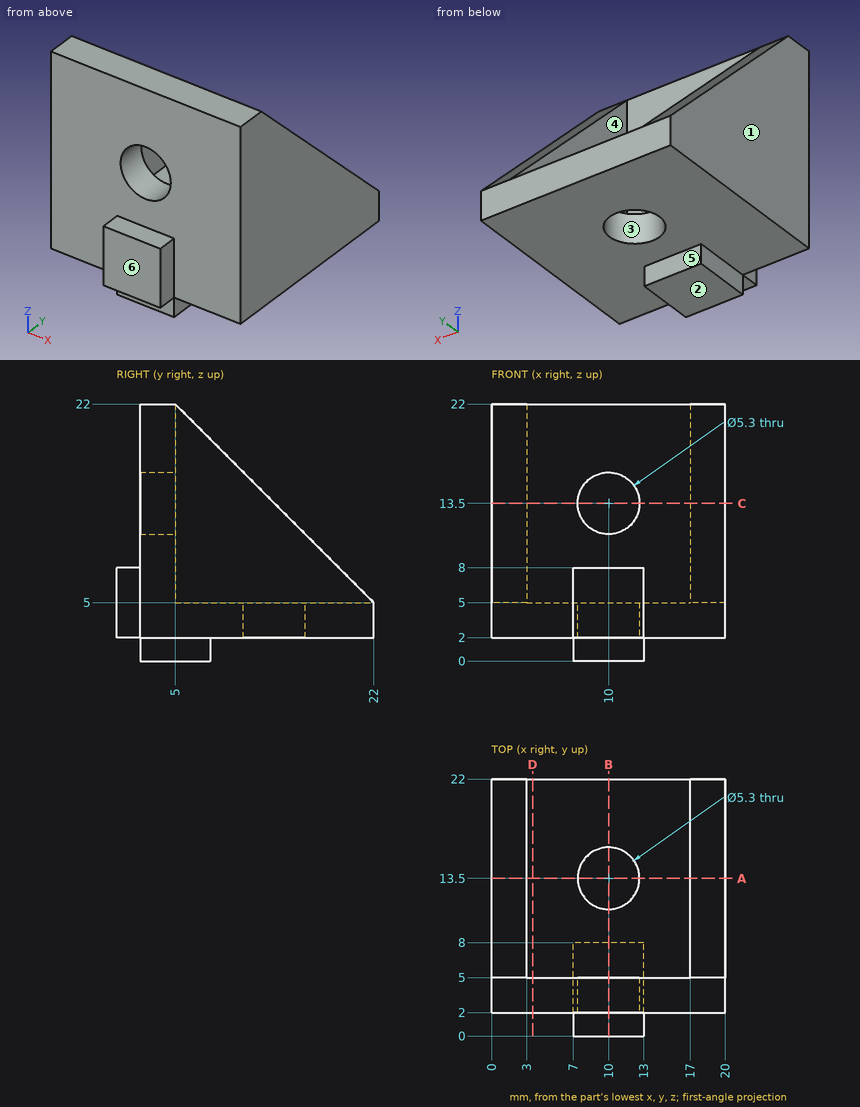
Could you check a few things on this drawing? It's one solid part, dimensions in mm from its lowest x, y, z. A direction names the side the tool comes from. Give positions to 0.01 mm unless a question says otherwise; leave off trailing zeros. Loops run counter-clockwise (first coordinate to the right, second up) from the corner with the lowest first, then second, coordinate; pieces in that order, holes last. Notation, with made-up numbers: (-29.5, 43) -> (-10.5, 43) arc R18 cw to (-10.5, 47) -> close; hole circle Ø9 at (80, 32.25). An arc over 180 degrees is marked (long way). Use one line per item in the form item = value. Start each with the question number.
1) Please list where these lines run through material, in increasing order: line 1 along X through (y, z) = (10.25, 14.5); line 2 along Y through (x, z) = (10, 4.15); line 3 along X through (y, z) = (3.55, 13.5).
2) Imagine slicing it at D-D (x = 3.5). Please give me the cut outline in (y, z), then the cut area to 3 significant figures.
3) Which directions (+Z, -Z, +X, -X, +Y, -Y) give clear straight access to the entire face, cutting with the end or side of a thin tool? Please do the marked faces 4, 5 and 6.
4) Thinking about a two-plate mould opening in X: for the marked faces 1, 2 and 3, which applies, +X half, -X half, draft (parallel to the pull), parting line (faces both ways), or undercut?
5) Imagine slicing it at B-B (x = 10). Please give me the cut outline in (y, z), then the cut area to 3 significant figures.
6) For P1, Ø0.6, axis at y = 1.5, z = 6, coming from the +X side; P2, Ø5, axis at x = 10, z = 13.5, coming from the +Y side; P3, Ø6, axis at x = 10, z = 14, coming from the -Y side; P4, Ø6, axis at x = 9.5, z = 13, coming from the +Y side, each with a flat end and sliding along its axis, tell me the tip position at first contact or that it passes through.
7) Imagine slicing it at A-A (y = 13.5). Please give me the cut outline in (x, z), then the cut area to 3 significant figures.
Check values:
q1.line_1 = 0 to 3, 17 to 20
q1.line_2 = 0 to 10.85, 16.15 to 22
q1.line_3 = 0 to 7.35, 12.65 to 20
q2.outline = (2, 2) -> (22, 2) -> (22, 5) -> (5, 5) -> (5, 22) -> (2, 22) -> close
q2.area = 111 mm^2
q3.face_4 = +Z, +Y
q3.face_5 = -Z, +X, -X, +Y
q3.face_6 = +Z, -Z, +X, -X, -Y
q4.face_1 = -X half
q4.face_2 = draft
q4.face_3 = undercut
q5.outline = (0, 2) -> (2, 2) -> (2, 0) -> (8, 0) -> (8, 2) -> (10.85, 2) -> (10.85, 5) -> (5, 5) -> (5, 10.85) -> (2, 10.85) -> (2, 8) -> (0, 8) -> close; (2, 16.15) -> (5, 16.15) -> (5, 22) -> (2, 22) -> close; (16.15, 2) -> (22, 2) -> (22, 5) -> (16.15, 5) -> close
q5.area = 103 mm^2
q6.P1 = 13
q6.P2 = through
q6.P3 = 2
q6.P4 = 5
q7.outline = (0, 2) -> (7.35, 2) -> (7.35, 5) -> (3, 5) -> (3, 13.5) -> (0, 13.5) -> close; (12.65, 2) -> (20, 2) -> (20, 13.5) -> (17, 13.5) -> (17, 5) -> (12.65, 5) -> close
q7.area = 95.1 mm^2
